The listing builds one solid part. Answer for the finished solid, in the listing's coordinates (mm). A direction names the side the tool comes from. Give positions to 0.01 mm unless a question says otherwise; leave off trailing zeros. Loops run counter-clockwise (first coordinate to the right, second up) from the corner with the lowest first, then second, coordinate; pieces in that order, holes last. Notation, with made-up numbers: (-1.75, -8.75) - (22.25, -8.75) arc R25 cw to (22.25, 13.25) - close; hole circle Ø3 at (75.5, 48.25). An arc over 180 degrees is marked (long way). Write item = value, one per line. Start each with the question number.
1) The part is cut by section B-B on y = 18.5. Write down the section's boundary in (x, z), plus the area to 4 significant figures.
2) Consider probe 1 along X at (y, z) = (2.15, -66.25); probe 2 along Z at (x, y) = (10.3, 0.6); probe 3 along X at (y, z) = (12.25, -59.5). Determine where each line is inside the solid, lowest interval first.
3) The part is cut by section A-A on x = 10.3. Write down the section's boundary in (y, z).
4) The part is cut by section D-D on x = 57. Write down the section's boundary in (y, z).
5) Flat-ended cylindrical pins translate along their axes: P1, Ø0.8, axis at x = 0.5, z = -22.5, coming from the +Y side; P2, Ø8.5, axis at x = 49.5, z = -31, coming from the +Y side; P3, Ø0.6, axis at x = 37.5, z = -26.5, coming from the +Y side. Find the tip coordinate at first contact, or state that the pin passes through.
6) The mould has two halves that part along X. Classify faces 1 (the flat face through (65, 3, -39)), 2 (the flat face through (39, 10, 0)), 3 (the flat face through (0, 6, -38)), 4 (the flat face through (46, 3, -39)): +X half, -X half, draft (parallel to the pull), parting line (faces both ways), or undercut.
7) The part is cut by section C-C on z = -40.5. Write down the section's boundary in (x, y), plus the area to 3 significant figures.
8) Which of the six approach directions +Z, -Z, +X, -X, +Y, -Y give full straight-line access (tool end or side, diameter ignored) to faces 5 (the flat face through (1, 13, -14)), 6 (the flat face through (39, 0, -39)), 7 (the flat face through (38.1, 8, -38))?
from build123d import *

# Parameters (mm, degrees)
SKETCH1_W             = 78.5
SKETCH1_H             = 77.5
BOSS_EXTRUDE1_DEPTH   = 21
SKETCH2_W             = 75.5
SKETCH2_H             = 74.5
CUT_EXTRUDE1_DEPTH    = 18
CUT_EXTRUDE2_DEPTH    = 113.292029993
RIB2_REACH            = 113.074
SKETCH5_WALLS_W       = 1.2
SKETCH5_WALLS_H       = 298.648598916
FILLET1_R             = 3
F_3_0MM_DOWEL_HOLE1_D = 3


with BuildPart() as part:
    # Sketch1 → Boss-Extrude1 (new body)
    with BuildSketch(Plane(origin=(0, 0, 0), x_dir=(1, 0, 0), z_dir=(0, 1, 0))):
        with Locations((39.25, 38.75)):
            Rectangle(SKETCH1_W, SKETCH1_H)
    extrude(amount=BOSS_EXTRUDE1_DEPTH)

    # Sketch2 → Cut-Extrude1 (cut)
    with BuildSketch(Plane(origin=(0, 21, 0), x_dir=(1, 0, 0), z_dir=(0, 1, 0))):
        with Locations((39.25, 38.75)):
            Rectangle(SKETCH2_W, SKETCH2_H)
    extrude(amount=-CUT_EXTRUDE1_DEPTH, mode=Mode.SUBTRACT)

    # Sketch3 → Cut-Extrude2 (cut, through all)
    with BuildSketch(Plane(origin=(78.5, 0, 0), x_dir=(0, 0, -1), z_dir=(1, 0, 0))):
        with BuildLine():
            Line((26, 7), (51.5, 7))
            Line((51.5, 7), (51.5, 10))
            ThreePointArc((51.5, 10), (51.792893219, 10.707106781), (52.5, 11))
            Line((52.5, 11), (61.085786438, 11))
            ThreePointArc((61.085786438, 11), (61.46846987, 11.076120467), (61.792893219, 11.292893219))
            Line((61.792893219, 11.292893219), (65.449747468, 14.949747468))
            ThreePointArc((65.449747468, 14.949747468), (65.774170817, 15.16652022), (66.156854249, 15.242640687))
            Line((66.156854249, 15.242640687), (76, 15.242640687))
            Line((76, 15.242640687), (76, 21))
            Line((76, 21), (1.5, 21))
            Line((1.5, 21), (1.5, 15.242640687))
            Line((1.5, 15.242640687), (11.343145751, 15.242640687))
            ThreePointArc((11.343145751, 15.242640687), (11.725829183, 15.16652022), (12.050252532, 14.949747468))
            Line((12.050252532, 14.949747468), (15.707106781, 11.292893219))
            ThreePointArc((15.707106781, 11.292893219), (16.03153013, 11.076120467), (16.414213562, 11))
            Line((16.414213562, 11), (25, 11))
            ThreePointArc((25, 11), (25.707106781, 10.707106781), (26, 10))
            Line((26, 10), (26, 7))
        make_face()
    extrude(amount=-CUT_EXTRUDE2_DEPTH, mode=Mode.SUBTRACT)

    # Sketch5 walls → Rib2 (add, up to next)
    with BuildSketch(Plane(origin=(0, 13, 0), x_dir=(1, 0, 0), z_dir=(0, 1, 0)), mode=Mode.PRIVATE) as rib2_sk1:
        with Locations((19.5, 38.75)):
            Rectangle(SKETCH5_WALLS_W, SKETCH5_WALLS_H)
    rib2_tool1 = extrude(rib2_sk1.sketch, amount=-RIB2_REACH, mode=Mode.PRIVATE) - part.part
    # Sketch5 walls → Rib2 (add, up to next)
    with BuildSketch(Plane(origin=(0, 13, 0), x_dir=(1, 0, 0), z_dir=(0, 1, 0)), mode=Mode.PRIVATE) as rib2_sk2:
        with Locations((37.5, 38.75)):
            Rectangle(SKETCH5_WALLS_W, SKETCH5_WALLS_H)
    rib2_tool2 = extrude(rib2_sk2.sketch, amount=-RIB2_REACH, mode=Mode.PRIVATE) - part.part
    # Sketch5 walls → Rib2 (add, up to next)
    with BuildSketch(Plane(origin=(0, 13, 0), x_dir=(1, 0, 0), z_dir=(0, 1, 0)), mode=Mode.PRIVATE) as rib2_sk3:
        with Locations((55.5, 38.75)):
            Rectangle(SKETCH5_WALLS_W, SKETCH5_WALLS_H)
    rib2_tool3 = extrude(rib2_sk3.sketch, amount=-RIB2_REACH, mode=Mode.PRIVATE) - part.part
    add(rib2_tool1.solids().sort_by_distance((19.5, 13, -38.75))[0])
    add(rib2_tool2.solids().sort_by_distance((37.5, 13, -38.75))[0])
    add(rib2_tool3.solids().sort_by_distance((55.5, 13, -38.75))[0])

    # Fillet1
    fillet1_edges = [part.edges().sort_by_distance(p)[0] for p in [
        (77, 3, -38.75),
        (1.5, 3, -38.75),
    ]]
    fillet(fillet1_edges, radius=FILLET1_R)

    # Ø3.0mm Dowel Hole1 (through all)
    with Locations(Plane(origin=(0, 0, 0), x_dir=(-1, 0, 0), z_dir=(0, -1, 0))):
        with Locations((-68.2, 11.25), (-48.9, 11.25), (-29.6, 11.25), (-10.3, 11.25), (-10.3, 66.25), (-29.6, 66.25), (-48.9, 66.25), (-68.2, 66.25)):
            Hole(F_3_0MM_DOWEL_HOLE1_D / 2)


solid = part.part
Answer below:
q1.outline = (0, -77.5) - (78.5, -77.5) - (78.5, -76) - (0, -76) - close; (0, -1.5) - (78.5, -1.5) - (78.5, 0) - (0, 0) - close
q1.area = 235.5 mm2
q2.probe_1 = 0 to 8.8, 11.8 to 28.1, 31.1 to 47.4, 50.4 to 66.7, 69.7 to 78.5
q2.probe_2 = -77.5 to -67.75, -64.75 to -12.75, -9.75 to 0
q2.probe_3 = 18.9 to 20.1, 36.9 to 38.1, 54.9 to 56.1
q3.outline = (0, -77.5) - (21, -77.5) - (21, -76) - (3, -76) - (3, -67.75) - (0, -67.75) - close; (0, -64.75) - (3, -64.75) - (3, -12.75) - (0, -12.75) - close; (0, -9.75) - (3, -9.75) - (3, -1.5) - (21, -1.5) - (21, 0) - (0, 0) - close
q4.outline = (0, -77.5) - (21, -77.5) - (21, -76) - (3, -76) - (3, -1.5) - (21, -1.5) - (21, 0) - (0, 0) - close
q5.P1 = 11
q5.P2 = 3
q5.P3 = 13
q6.face_1 = undercut
q6.face_2 = draft
q6.face_3 = -X half
q6.face_4 = undercut
q7.outline = (0, 0) - (78.5, 0) - (78.5, 7) - (77, 7) - (77, 6) arc R3 cw to (74, 3) - (56.1, 3) - (56.1, 13) - (54.9, 13) - (54.9, 3) - (38.1, 3) - (38.1, 13) - (36.9, 13) - (36.9, 3) - (20.1, 3) - (20.1, 13) - (18.9, 13) - (18.9, 3) - (4.5, 3) arc R3 cw to (1.5, 6) - (1.5, 7) - (0, 7) - close
q7.area = 287 mm2
q8.face_5 = -X, +Y
q8.face_6 = +Z, -Z, +X, -X, -Y
q8.face_7 = +Y
